from build123d import *

# Parameters (mm, degrees)
PAD_DEPTH       = 4
SKETCH001_R     = 2.6
PAD001_DEPTH    = 5
SKETCH002_R     = 2.15
POCKET_DEPTH    = 4.001
SKETCH003_W     = 6.3
SKETCH003_H     = 6.3
POCKET001_DEPTH = 2.5
FILLET_R        = 4
CHAMFER_SIZE    = 1
SKETCH004_R     = 4.65
POCKET002_DEPTH = 4.001
FILLET001_R     = 3


with BuildPart() as part:
    # Sketch → Pad (new body)
    with BuildSketch(Plane.XY):
        with BuildLine():
            ThreePointArc((-10.894444, -35.359738), (0, -37), (10.894444, -35.359738))
            ThreePointArc((13.25, -51.005087), (21.16084, -41.814035), (10.894444, -35.359738))
            Line((13.25, -51.005087), (5, -51.005087))
            Line((5, -51.005087), (5, -86.005087))
            Line((-5, -86.005087), (5, -86.005087))
            Line((-5, -51.005087), (-5, -86.005087))
            Line((-13.25, -51.005087), (-5, -51.005087))
            ThreePointArc((-10.894444, -35.359738), (-21.16084, -41.814035), (-13.25, -51.005087))
        make_face()
    extrude(amount=PAD_DEPTH)

    # Sketch001 (on Face10 of Pad) → Pad001 (join)
    with BuildSketch(Plane.XY.offset(4)):
        with Locations((-13.25, -43.005087)):
            Circle(SKETCH001_R)
        with Locations((13.25, -43.005087)):
            Circle(SKETCH001_R)
    extrude(amount=PAD001_DEPTH)

    # Sketch002 (on Face5 of Pad001) → Pocket (cut, through all)
    with BuildSketch(Plane.XY.offset(4)):
        with Locations((0, -43.505087)):
            Circle(SKETCH002_R)
        with Locations((0, -78.005087)):
            Circle(SKETCH002_R)
    extrude(amount=-POCKET_DEPTH, mode=Mode.SUBTRACT)

    # Sketch003 (on Face5 of Pocket) → Pocket001 (cut)
    with BuildSketch(Plane.XY.offset(4)):
        with Locations((0, -43.505087)):
            Rectangle(SKETCH003_W, SKETCH003_H)
        with Locations((0, -78.005087)):
            Rectangle(SKETCH003_W, SKETCH003_H)
    extrude(amount=-POCKET001_DEPTH, mode=Mode.SUBTRACT)

    # Fillet
    fillet_edges = [part.edges().sort_by_distance(p)[0] for p in [
        (5, -51.005087, 2),
        (-5, -51.005087, 2),
        (-5, -86.005087, 2),
        (5, -86.005087, 2),
    ]]
    fillet(fillet_edges, radius=FILLET_R)

    # Chamfer
    chamfer_edges = [part.edges().sort_by_distance(p)[0] for p in [
        (-15.85, -43.005087, 9),
        (10.65, -43.005087, 9),
    ]]
    chamfer(chamfer_edges, length=CHAMFER_SIZE)

    # Sketch004 (on Face3 of Chamfer) → Pocket002 (cut, through all)
    with BuildSketch(Plane.XY.offset(4)):
        with Locations((-7, -60.755087)):
            Circle(SKETCH004_R)
    extrude(amount=-POCKET002_DEPTH, mode=Mode.SUBTRACT)

    # Fillet001
    fillet001_edges = [part.edges().sort_by_distance(p)[0] for p in [
        (-5, -56.557171, 2),
        (-5, -64.953003, 2),
    ]]
    fillet(fillet001_edges, radius=FILLET001_R)


solid = part.part
The listing builds one solid part. Answer for the finished solid, in the listing's coordinates (mm). A direction names the side the tool comes from. Round coordinates to 2 decimals unless told otherwise and drop trailing zeros. Write each loop counter-clockwise with the first axis right and the second up, starting at its lowest first coordinate (ties: lowest second). Pieces come first, ordered by that corner, then holes. Notation, with made-up numbers: M 67.5,4.5 L 122.5,4.5 A25 cw 122.5,38.5 Z; hole C -23.75,27 d5. An arc over 180 degrees is marked long. Write each question's results on one line, items separated by ' | '. Start each with the question number.
Item 1: Which of the six approach directions +Z, -Z, +X, -X, +Y, -Y give full straight-line access (tool end or side, diameter ignored) to faces 4 (the flat face through (0, -86.005, 2)), 5 (the flat face through (3.15, -78, 3)), 6 (the flat face through (-5, -74, 2))?
Item 2: Find section B-B on z = 2.25. Give the number of separate pieces and of enclosed holes in the cut face, and give its area (3 significant figures).
Item 3: The mould has two halves that part along Y. Classify faces 1 (the flat face through (-13, -43, 9)), 2 (the cylindrical face through (21.187, -42.005, 1.972)), 3 (the flat face through (0, -74.855, 3)): +Y half, -Y half, draft (parallel to the pull), parting line (faces both ways), or undercut.
Item 4: Find section A-A on x = 0. Write down the section's boundary in (y, z).
Item 5: Straight lines are drawn through the part: probe 1 along Y at (x, z) = (0, 0.3); probe 2 along Z at (x, y) = (8, -37.5); probe 3 along X at (y, z) = (-46.5, 2.25). For each, find the intervals that lie inside material, in ascending order.
Item 6: Find section D-D on x = -10. Write down the section's boundary in (y, z), and give its area (3 significant figures).
Item 7: Find section C-C on y = -68. Write down the section's boundary in (x, z).
Item 8: Given pin 1 Ø1.9 at (x, y) = (0.5, -44) entering from +Z; pin 2 Ø2 at (x, z) = (10, 1.5) entering from -Y; pin 3 Ø7 at (x, y) = (-0.5, -77.5) entering from +Z; pin 4 Ø1.2 at (y, z) = (-77, 3) entering from +X, each flat-ended and moving along its own axis, determine where each tip first touches the part or whether it passes through.
Answer block:
1) face 4: +Z, -Z, +X, -X, -Y | face 5: +Z | face 6: +Z, -Z, -X, -Y
2) separate pieces: 1 | enclosed holes: 2 | area: 847 mm²
3) face 1: draft | face 2: parting line | face 3: undercut
4) outline: M -86.01,0 L -80.16,0 L -80.16,1.5 L -81.16,1.5 L -81.16,4 L -86.01,4 Z; M -75.86,0 L -45.66,0 L -45.66,1.5 L -46.66,1.5 L -46.66,4 L -74.86,4 L -74.86,1.5 L -75.86,1.5 Z; M -41.36,0 L -37,0 L -37,4 L -40.36,4 L -40.36,1.5 L -41.36,1.5 Z
5) probe 1: y = -86.01 to -80.16, -75.86 to -45.66, -41.36 to -37 | probe 2: z = 0 to 4 | probe 3: x = -20.45 to -3.15, 3.15 to 20.45
6) outline: M -51.01,0 L -35.62,0 L -35.62,4 L -51.01,4 Z | area: 61.5 mm²
7) outline: M -5,0 L 5,0 L 5,4 L -5,4 Z
8) pin 1: passes through | pin 2: stops at y = -51.01 | pin 3: stops at z = 4 | pin 4: stops at x = 5
